from build123d import *

# Parameters (mm, degrees)
BOSS_EXTRUDE1_DEPTH = 304.8
SKETCH3_R           = 4.7625
CUT_EXTRUDE2_DEPTH  = 76.2


with BuildPart() as part:
    # Sketch1 → Boss-Extrude1 (new, symmetric)
    with BuildSketch(Plane.XY):
        with BuildLine():
            Line((-19.685, 25.4), (19.685, 25.4))
            ThreePointArc((19.685, 25.4), (23.726115254, 23.726115254), (25.4, 19.685))
            Line((25.4, 19.685), (25.4, -19.685))
            ThreePointArc((25.4, -19.685), (23.726115254, -23.726115254), (19.685, -25.4))
            Line((19.685, -25.4), (-19.685, -25.4))
            ThreePointArc((-19.685, -25.4), (-23.726115254, -23.726115254), (-25.4, -19.685))
            Line((-25.4, -19.685), (-25.4, 19.685))
            ThreePointArc((-25.4, 19.685), (-23.726115254, 23.726115254), (-19.685, 25.4))
        make_face()
        with BuildLine():
            Line((-19.685, -22.225), (19.685, -22.225))
            ThreePointArc((19.685, -22.225), (21.481051224, -21.481051224), (22.225, -19.685))
            Line((22.225, -19.685), (22.225, 19.685))
            ThreePointArc((22.225, 19.685), (21.481051224, 21.481051224), (19.685, 22.225))
            Line((19.685, 22.225), (-19.685, 22.225))
            ThreePointArc((-19.685, 22.225), (-21.481051224, 21.481051224), (-22.225, 19.685))
            Line((-22.225, 19.685), (-22.225, -19.685))
            ThreePointArc((-22.225, -19.685), (-21.481051224, -21.481051224), (-19.685, -22.225))
        make_face(mode=Mode.SUBTRACT)
    extrude(amount=BOSS_EXTRUDE1_DEPTH, both=True)

    # Sketch3 → Cut-Extrude2 (cut)
    with BuildSketch(Plane(origin=(25.4, 0, 0), x_dir=(0, 0, -1), z_dir=(1, 0, 0))):
        with Locations(Location((50.8, 0, 0), (0, 0, 90))):
            Circle(SKETCH3_R)
    extrude(amount=-CUT_EXTRUDE2_DEPTH, mode=Mode.SUBTRACT)


solid = part.part
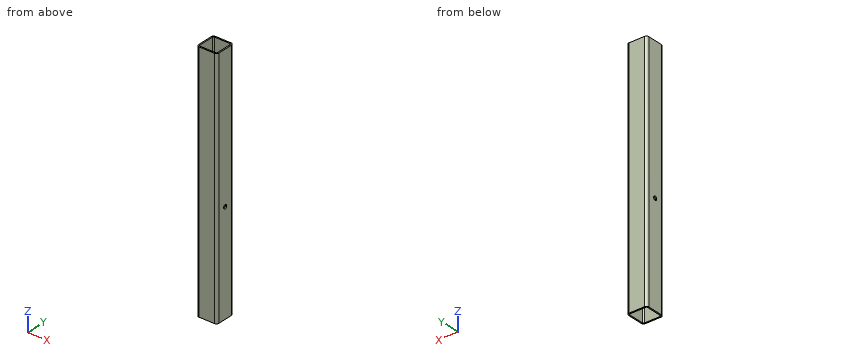
The model under review builds one solid part; all positions refer to its coordinate system, in mm. Give positions to 0.01 mm unless a question says otherwise; leave off trailing zeros. Write each loop counter-clockwise with the first axis right and the second up, starting at its lowest first coordinate (ties: lowest second). Pieces come first, ordered by that corner, then holes. Notation, with made-up numbers: M 87,24 L 92,24 A20 cw 92,58 Z; hole C 13,67.25 d2. An arc over 180 degrees is marked long. One line per question, with ' | ' between items. Start each with the question number.
Item 1: Wall thickness on line 1 (X direction, y = 20, z = 5.5); line 2 (Z direction, x = 24.55, y = 0); line 3 (Y direction, x = 2, z = -38.5) (3 decimals): over which ranges is each line inside the solid? List them lowest first. Write a range as from..to.
Item 2: For pin 1 (8 mm diameter, centred on x = 12.5, y = -16.5, fed in from -Z), flat-tipped, find the tip position at first contact; note if it passes through.
Item 3: We need section C-C on z = -196.5. Write out the cut boundary in (x, y) (3 decimals), plus the area to 3 significant figures.
Item 4: We need section A-A on x = -13. Write out the cut boundary in (y, z) (3 decimals), plus the area to 3 significant figures.
Results found:
1) line 1: x = -25.39..-22.21, 22.21..25.39 | line 2: z = -304.8..-55.56, -46.04..304.8 | line 3: y = -25.4..-22.225, 22.225..25.4
2) pin 1: passes through
3) outline: M -25.4,-19.685 A5.715 ccw -19.685,-25.4 L 19.685,-25.4 A5.715 ccw 25.4,-19.685 L 25.4,19.685 A5.715 ccw 19.685,25.4 L -19.685,25.4 A5.715 ccw -25.4,19.685 Z; hole M -22.225,-19.685 A2.54 ccw -19.685,-22.225 L 19.685,-22.225 A2.54 ccw 22.225,-19.685 L 22.225,19.685 A2.54 ccw 19.685,22.225 L -19.685,22.225 A2.54 ccw -22.225,19.685 Z | area: 582 mm2
4) outline: M -25.4,-304.8 L -22.225,-304.8 L -22.225,304.8 L -25.4,304.8 Z; M 22.225,-304.8 L 25.4,-304.8 L 25.4,304.8 L 22.225,304.8 Z | area: 3,870 mm2
